Model file for the job. Use its own axes, mm. Face numbers are marked on the shaded views. A direction names the side the tool comes from. Coordinates: 2 decimals unless noted, no trailing zeros. Order: outer loops, then holes, each group sorted by start corner. A loop starts at its lowest first (then second) coordinate and runs counter-clockwise, first axis right, second up.
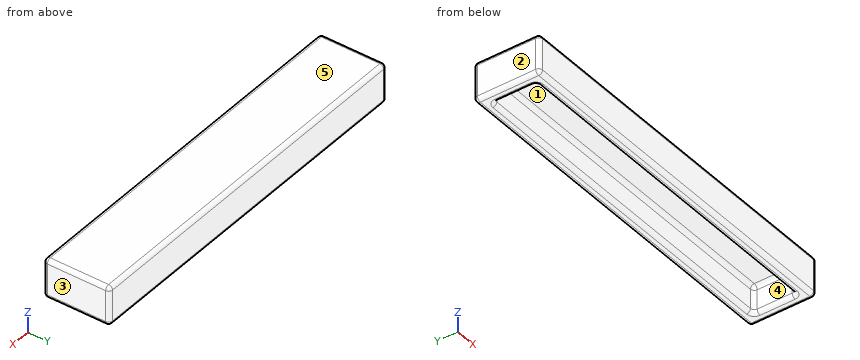
from build123d import *

# Parameters (mm, degrees)
F0_W     = 95
F0_H     = 17
F1_DEPTH = 10
F2_T     = -3
F3_R     = 1


with BuildPart() as f1:
    # F0 (on Top) → F1 (new body)
    with BuildSketch(Plane.XY):
        with Locations((-0.1398691535, -5.5)):
            Rectangle(F0_W, F0_H)
    extrude(amount=F1_DEPTH)

    # F2
    f2_openings = [f1.faces().sort_by_distance(p)[0] for p in [
        (-0.139869, -5.5, 0),
    ]]
    offset(amount=F2_T, openings=f2_openings)

    # F3
    f3_edges = [f1.edges().sort_by_distance(p)[0] for p in [
        (-44.639869, -5.5, 7),
        (-0.139869, -11, 7),
        (44.360131, -5.5, 7),
        (-0.139869, 0, 7),
        (-0.139869, 0, 0),
        (44.360131, 0, 3.5),
        (-44.639869, 0, 3.5),
        (-0.139869, -11, 0),
        (-44.639869, -11, 3.5),
        (44.360131, -11, 3.5),
        (47.360131, -14, 5),
        (47.360131, 3, 5),
        (47.360131, -5.5, 0),
        (47.360131, -5.5, 10),
        (-47.639869, -14, 5),
        (-0.139869, -14, 0),
        (-0.139869, -14, 10),
        (-47.639869, 3, 5),
        (-0.139869, 3, 0),
        (-0.139869, 3, 10),
        (-47.639869, -5.5, 0),
        (-47.639869, -5.5, 10),
        (44.360131, -5.5, 0),
        (-44.639869, -5.5, 0),
    ]]
    fillet(f3_edges, radius=F3_R)


solid = f1.part
Q1. Cut at A-A, the plane z = 3.75. List the corners of the cut face in (x, y), plus the area to 3 significant figures.
Established:
outline: (-47.64, -13) arc R1 ccw to (-46.64, -14) - (46.36, -14) arc R1 ccw to (47.36, -13) - (47.36, 2) arc R1 ccw to (46.36, 3) - (-46.64, 3) arc R1 ccw to (-47.64, 2) - close; hole (-44.64, -10) arc R1 ccw to (-43.64, -11) - (43.36, -11) arc R1 ccw to (44.36, -10) - (44.36, -1) arc R1 ccw to (43.36, 0) - (-43.64, 0) arc R1 ccw to (-44.64, -1) - close
area: 636 mm2
Q2. Which spindle directions (+Z, -Z, +X, -X, +Y, -Y) get a long thin tool onto all of the face, cutting with end or side? Do the marked faces 1 and 2. Say none if no direction does.
Established:
face 1: -Z
face 2: +Z, -Z, -X, +Y, -Y
Q3. Cut at C-C, the plane y = -6.25. List the corners of the cut face in (x, z).
Established:
outline: (-47.64, 1) arc R1 ccw to (-46.64, 0) - (-45.64, 0) arc R1 ccw to (-44.64, 1) - (-44.64, 6) arc R1 cw to (-43.64, 7) - (43.36, 7) arc R1 cw to (44.36, 6) - (44.36, 1) arc R1 ccw to (45.36, 0) - (46.36, 0) arc R1 ccw to (47.36, 1) - (47.36, 9) arc R1 ccw to (46.36, 10) - (-46.64, 10) arc R1 ccw to (-47.64, 9) - close
Q4. Cut at B-B, the plane x = -24.5. List the corners of the cut face in (y, z).
Established:
outline: (-14, 1) arc R1 ccw to (-13, 0) - (-12, 0) arc R1 ccw to (-11, 1) - (-11, 6) arc R1 cw to (-10, 7) - (-1, 7) arc R1 cw to (0, 6) - (0, 1) arc R1 ccw to (1, 0) - (2, 0) arc R1 ccw to (3, 1) - (3, 9) arc R1 ccw to (2, 10) - (-13, 10) arc R1 ccw to (-14, 9) - close
Q5. Drop a flat-ended pin along its axis: P1, Ø6, axis at x = 5, y = -4, coming from the -Z side. Give the stop position or say it passes through.
Established:
P1: stops at z = 7
Q6. Probe line 1 (X direction, y = -6, z = 3); line 2 (Y direction, x = -7, z = 3.75); line 3 (Z direction, x = 10, y = -8.25). List the from-to ranges inside material, lowest first.
Established:
line 1: x = -47.64 to -44.64, 44.36 to 47.36
line 2: y = -14 to -11, 0 to 3
line 3: z = 7 to 10
Q7. Mould opens along X. For the marked faces 3, 4 and 5 say: pulls with the +X half, pulls with the -X half, needs draft (parallel to the pull), parting line crosses it, or undercut.
Established:
face 3: pulls with the +X half
face 4: undercut
face 5: needs draft
